The listing builds one solid part. Answer for the finished solid, in the listing's coordinates (mm). Face numbers are marked on the shaded views. Coordinates: 2 decimals unless noted, no trailing zeros. Order: outer loops, then holes, each group sorted by start corner. A loop starts at its lowest first (then second) coordinate and runs counter-clockwise, first axis right, second up.
```python
from build123d import *


with BuildPart() as part:
    # Szkic2 → Obrót1 (revolve)
    with BuildSketch(Plane.XY, mode=Mode.PRIVATE) as obr_t1_sk:
        Polygon((-425.537809827, -177.948573753), (-422.037809827, -177.948573753), (-422.037809827, -178.148573753), (-419.037809827, -178.148573753), (-419.037809827, -177.948573753), (-415.537809827, -177.948573753), (-415.537809827, -179.448573753), (-425.537809827, -179.448573753), align=None)
    revolve(obr_t1_sk.sketch.rotate(Axis((-411.49910078, -202.948573753, 0), (1, 0, 0)), 90), axis=Axis((-411.49910078, -202.948573753, 0), (1, 0, 0)))


solid = part.part
```
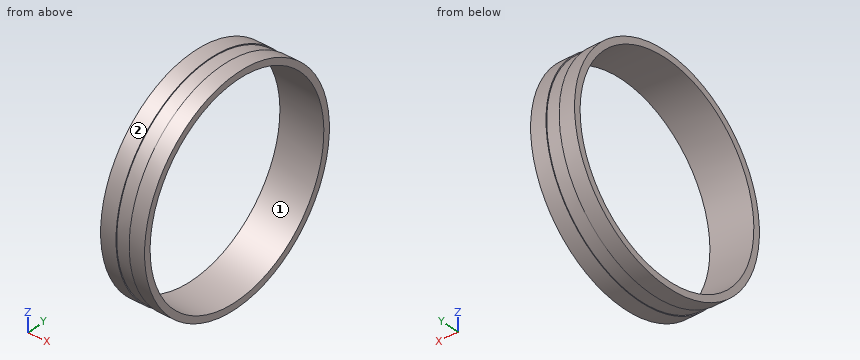
(1) Find section B-B (y = -218). Write down the section's boundary in (x, z).
(2) Find section C-C (x = -420). Write down the section's boundary in (y, z), and give its area (3 significant figures).
(3) Consider line 1 (X direction, y = -188, z = 20); line 2 (Y direction, x = -419.5, z = 0); line 3 (Y direction, x = -418.5, z = 0). Determine where each line is inside the solid, lowest interval first.
(4) Find section D-D (x = -424.5). Write down the section's boundary in (y, z), and give its area (3 significant figures).
(5) Each of these flat-tipped pins is pushed along its axis until it touches: pin 1 Ø6 at (x, y) = (-420, -208.5) entering from -Z; pin 2 Ø4 at (x, z) = (-424, -8.5) entering from +Y; pin 3 Ø4 at (x, z) = (-420.5, -13.5) entering from +Y; pin 4 Ø8 at (y, z) = (-192.5, 16) entering from +X. Where does it stop, or does it pass through?
(6) The mould has two halves that part along Z. Classify the marked faces 1 and 2: released by +Z, released by -Z, zero draft, split by the parting line, or undercut.
(7) Find section A-A (z = 0). Write down the section's boundary in (x, y).
Findings below:
1. outline: (-425.54, -19.96) - (-422.04, -19.96) - (-422.04, -19.71) - (-419.04, -19.71) - (-419.04, -19.96) - (-415.54, -19.96) - (-415.54, -18.05) - (-425.54, -18.05) - close; (-425.54, 18.05) - (-415.54, 18.05) - (-415.54, 19.96) - (-419.04, 19.96) - (-419.04, 19.71) - (-422.04, 19.71) - (-422.04, 19.96) - (-425.54, 19.96) - close
2. outline: circle Ø49.6 at (-202.95, 0); hole circle Ø47 at (-202.95, 0)
2. area: 197 mm2
3. line 1: x = -425.54 to -422.04, -419.04 to -415.54
3. line 2: y = -227.75 to -226.45, -179.45 to -178.15
3. line 3: y = -227.95 to -226.45, -179.45 to -177.95
4. outline: circle Ø50 at (-202.95, 0); hole circle Ø47 at (-202.95, 0)
4. area: 229 mm2
5. pin 1: stops at z = -24.85
5. pin 2: stops at y = -178.81
5. pin 3: stops at y = -180.98
5. pin 4: passes through
6. face 1: undercut
6. face 2: split by the parting line
7. outline: (-425.54, -227.95) - (-422.04, -227.95) - (-422.04, -227.75) - (-419.04, -227.75) - (-419.04, -227.95) - (-415.54, -227.95) - (-415.54, -226.45) - (-425.54, -226.45) - close; (-425.54, -179.45) - (-415.54, -179.45) - (-415.54, -177.95) - (-419.04, -177.95) - (-419.04, -178.15) - (-422.04, -178.15) - (-422.04, -177.95) - (-425.54, -177.95) - close
